from build123d import *

# Parameters (mm, degrees)
SKETCH1_W           = 38
SKETCH1_H           = 4.8
BOSS_EXTRUDE1_DEPTH = 38
SKETCH2_R           = 2
CUT_EXTRUDE1_DEPTH  = 10
SKETCH3_R           = 6
CUT_EXTRUDE2_DEPTH  = 5.8


with BuildPart() as part:
    # Sketch1 → Boss-Extrude1 (new body)
    with BuildSketch(Plane(origin=(0, 0, 0), x_dir=(1, 0, 0), z_dir=(0, 1, 0))):
        Rectangle(SKETCH1_W, SKETCH1_H)
    extrude(amount=BOSS_EXTRUDE1_DEPTH)

    # Sketch2 → Cut-Extrude1 (cut)
    with BuildSketch(Plane.XZ):
        with Locations((7.75, 0)):
            Circle(SKETCH2_R)
        with Locations((-7.75, 0)):
            Circle(SKETCH2_R)
    extrude(amount=-CUT_EXTRUDE1_DEPTH, mode=Mode.SUBTRACT)

    # Sketch3 → Cut-Extrude2 (cut, through all)
    with BuildSketch(Plane.XY.offset(2.4)):
        with Locations((-7, 19)):
            Circle(SKETCH3_R)
    extrude(amount=-CUT_EXTRUDE2_DEPTH, mode=Mode.SUBTRACT)


solid = part.part
Work out the finished part from the listing and answer in its coordinate system (mm). A direction names the side the tool comes from. Coordinates: 2 decimals unless noted, no trailing zeros. Order: outer loops, then holes, each group sorted by start corner. A loop starts at its lowest first (then second) coordinate and runs counter-clockwise, first axis right, second up. Notation, with made-up numbers: (-26, 61.25) - (3, 61.25) arc R28 cw to (3, 85.25) - close; hole circle Ø4 at (16, 68). An arc over 180 degrees is marked (long way). Put each result on its own line as item: value. Start each with the question number.
1) Find section A-A (y = 18.5). Give the vertices of the cut face in (x, z).
2) For faces 4 (the cylindrical face through (-9.748, 4.93, 0.088)), 5 (the flat face through (-19, 19, 0)), determine the directions among +Z, -Z, +X, -X, +Y, -Y from which every point of the face is accessible in a straight line to the end or side of a thin tool.
3) Find section B-B (x = -7.75). Give the vertices of the cut face in (y, z), plus the area to 3 significant figures.
4) Find the intervals of material crossed by line 1 (Y direction, x = -7, z = 0); line 2 (Z direction, x = 7.75, y = 2.5); line 3 (X direction, y = 2.5, z = -1.3), in increasing order. Write a range as from..to.
5) For a pull along Z with two mould halves and no side action, classify faces 1 (the flat face through (-8, 10, 0)), 2 (the flat face through (19, 19, 0)), 3 (the flat face through (0, 19, -2.4)) as released by +Z, released by -Z, zero draft, split by the parting line, or undercut.
6) Find section C-C (z = -1.1). Give the vertices of the cut face in (x, y).
7) Find section D-D (y = 5). Give the vertices of the cut face in (x, z).
Results list:
1. outline: (-19, -2.4) - (-12.98, -2.4) - (-12.98, 2.4) - (-19, 2.4) - close; (-1.02, -2.4) - (19, -2.4) - (19, 2.4) - (-1.02, 2.4) - close
2. face 4: -Y
2. face 5: +Z, -Z, -X, +Y, -Y
3. outline: (0, -2.4) - (13.05, -2.4) - (13.05, 2.4) - (0, 2.4) - (0, 2) - (10, 2) - (10, -2) - (0, -2) - close; (24.95, -2.4) - (38, -2.4) - (38, 2.4) - (24.95, 2.4) - close
3. area: 85.3 mm^2
4. line 1: y = 10..13, 25..38
4. line 2: z = -2.4..-2, 2..2.4
4. line 3: x = -19..-9.27, -6.23..6.23, 9.27..19
5. face 1: undercut
5. face 2: zero draft
5. face 3: released by -Z
6. outline: (-19, 0) - (-9.42, 0) - (-9.42, 10) - (-6.08, 10) - (-6.08, 0) - (6.08, 0) - (6.08, 10) - (9.42, 10) - (9.42, 0) - (19, 0) - (19, 38) - (-19, 38) - close; hole circle Ø12 at (-7, 19)
7. outline: (-19, -2.4) - (19, -2.4) - (19, 2.4) - (-19, 2.4) - close; hole circle Ø4 at (-7.75, 0); hole circle Ø4 at (7.75, 0)
